```python
from build123d import *

# Parameters (mm, degrees)
SKETCH1_R           = 7.7
BOSS_EXTRUDE3_DEPTH = 102.14
BOSS_EXTRUDE3_DRAFT = -0.2
SKETCH3_R           = 6.25
SKETCH3_R_2         = 6.1
BOSS_EXTRUDE4_DEPTH = 4.6
CHAMFER1_SIZE       = 0.6
CHAMFER1_SIZE2      = 5
FILLET1_R           = 0.5
FILLET2_R           = 10
CHAMFER2_SIZE       = 0.3
CHAMFER2_SIZE2      = 0.1


with BuildPart() as part:
    # Sketch1 → Boss-Extrude3 (with draft: the straight prism first)
    with BuildSketch(Plane.XY):
        Circle(SKETCH1_R)
    extrude(amount=-BOSS_EXTRUDE3_DEPTH)
    # Boss-Extrude3: the draft: its side faces are tilted about the plane it starts from
    boss_extrude3_sides = [part.faces().sort_by_distance(p)[0] for p in [
        (-7.7, 0, -51.07),
    ]]
    draft(boss_extrude3_sides, Plane.XY, BOSS_EXTRUDE3_DRAFT)

    # Sketch3 → Boss-Extrude4 (add)
    with BuildSketch(Plane.XY):
        Circle(SKETCH3_R)
        Circle(SKETCH3_R_2, mode=Mode.SUBTRACT)
    extrude(amount=BOSS_EXTRUDE4_DEPTH)

    # Chamfer1
    chamfer1_edges = [part.edges().sort_by_distance(p)[0] for p in [
        (-7.343462692, 0, -102.14),
    ]]
    chamfer1_side = [part.faces().sort_by_distance(p)[0] for p in [
        (0, 0, -102.14),
    ]]
    chamfer(chamfer1_edges, length=CHAMFER1_SIZE, length2=CHAMFER1_SIZE2, reference=chamfer1_side[0])

    # Fillet1
    fillet1_edges = [part.edges().sort_by_distance(p)[0] for p in [
        (-6.743462692, 0, -102.14),
    ]]
    fillet(fillet1_edges, radius=FILLET1_R)

    # Fillet2
    fillet2_edges = [part.edges().sort_by_distance(p)[0] for p in [
        (-7.360915949, 0, -97.140030462),
    ]]
    fillet(fillet2_edges, radius=FILLET2_R)

    # Chamfer2
    chamfer2_edges = [part.edges().sort_by_distance(p)[0] for p in [
        (-6.25, 0, 4.6),
    ]]
    chamfer2_side = [part.faces().sort_by_distance(p)[0] for p in [
        (-6.25, 0, 2.3),
    ]]
    chamfer(chamfer2_edges, length=CHAMFER2_SIZE, length2=CHAMFER2_SIZE2, reference=chamfer2_side[0])


solid = part.part
```
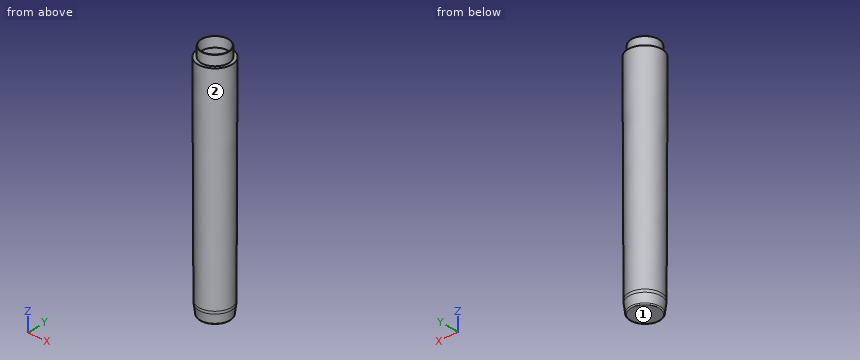
Check sheet for the modelled part. Datum: model origin and axes. Units: mm. Face numbers are marked on the shaded views. A direction names the side the tool comes from. Coordinates: 2 decimals unless noted, no trailing zeros. Order: outer loops, then holes, each group sorted by start corner. A loop starts at its lowest first (then second) coordinate and runs counter-clockwise, first axis right, second up. Notation, with made-up numbers: M 36.25,39.25 L 46.25,39.25 A15 ccw 46.25,57.25 Z; hole C -25,40 d11. An arc over 180 degrees is marked long. Write each question's results on one line, items separated by ' | '. Start each with the question number.
1. Access from +Z, -Z, +X, -X, +Y, -Y to the whole of each face (thin tool, end or side, straight path). Record for the marked faces 1 and 2.
2. Material ranges on probe 1 along Z at (x, y) = (-4, 2.75); probe 2 along Y at (x, z) = (1.75, -40.5); probe 3 along X at (y, z) = (0.75, -3.5), recorded low to high.
3. Cross-section at B-B on z = -51.5. Record the cut outline in (x, y).
4. Cross-section at A-A on z = -67. Record the cut outline in (x, y).
5. Go/stop test with flat-tipped pins: P1, Ø3, axis at x = 0, z = -35.5, coming from the +Y side; P2, Ø6, axis at x = -1.5, z = -83, coming from the +Y side; P3, Ø2, axis at y = 2, z = -77.5, coming from the -X side. Record where each tip stops, or that it passes through.
Checks:
1) face 1: -Z, +X, -X, +Y, -Y | face 2: -Z
2) probe 1: z = -102.14 to 0 | probe 2: y = -7.35 to 7.35 | probe 3: x = -7.65 to 7.65
3) outline: C 0,0 d15.04
4) outline: C 0,0 d14.93
5) P1: stops at y = 7.58 | P2: stops at y = 7.42 | P3: stops at x = -7.36
